Source: CAD feature listing. Evaluate the final solid. Frame: model axes, mm. A direction names the side the tool comes from. Coordinates: 2 decimals unless noted, no trailing zeros. Order: outer loops, then holes, each group sorted by start corner. A loop starts at its lowest first (then second) coordinate and runs counter-clockwise, first axis right, second up.
```python
from build123d import *

# Parameters (mm, degrees)
SKETCH2_W                      = 198.000030872
SKETCH2_H                      = 103.32125718
CUT_EXTRUDE1_DEPTH             = 3.6
FILLET1_R                      = 5
FILLET2_R                      = 3
F_4_CLEARANCE_HOLE1_AT_2_COUNT = 2
F_4_CLEARANCE_HOLE1_AT_2_PITCH = 13
CIRPATTERN1_COUNT              = 4
CIRPATTERN1_ANGLE              = 165
CUT_EXTRUDE2_DEPTH             = 3.6000001


with BuildPart() as part:
    # Sketch1 → Revolve1 (revolve)
    with BuildSketch(Plane(origin=(0, 0, 0), x_dir=(0, 0, -1), z_dir=(1, 0, 0)), mode=Mode.PRIVATE) as revolve1_sk:
        Polygon((0, 22), (0, 63), (1.5, 63), (1.5, 35), (2.6, 32.5), (2.6, 22), align=None)
    revolve(revolve1_sk.sketch.rotate(Axis((0, 0, 0), (0, 0, -1)), 90), axis=Axis((0, 0, 0), (0, 0, -1)))  # turned: the seam where the file's is

    # Sketch2 → Cut-Extrude1 (cut, through all)
    with BuildSketch(Plane.XY):
        with Locations((-0.69062002, -48.66062859)):
            Rectangle(SKETCH2_W, SKETCH2_H)
    extrude(amount=-CUT_EXTRUDE1_DEPTH, mode=Mode.SUBTRACT)

    # Fillet1
    fillet1_edges = [part.edges().sort_by_distance(p)[0] for p in [
        (0, 32.5, -2.6),
        (0, 35, -1.5),
    ]]
    fillet(fillet1_edges, radius=FILLET1_R)

    # Fillet2
    fillet2_edges = [part.edges().sort_by_distance(p)[0] for p in [
        (-21.794494718, 3, -1.3),
        (-62.92853089, 3, -0.75),
        (21.794494718, 3, -1.3),
        (62.92853089, 3, -0.75),
    ]]
    fillet(fillet2_edges, radius=FILLET2_R)

    # Sketch3 → #4 Clearance Hole1 (revolve, cut)
    with BuildSketch(Plane(origin=(-59.486691682, 7.831571533, 0), x_dir=(0, -1, 0), z_dir=(1, 0, 0))):
        Polygon((0, 0), (0, 136.775187864), (1.4732, 135.89), (1.4732, 0), align=None)
    f_4_clearance_hole1 = revolve(axis=Axis((-59.486691682, 7.831571533, 6.35), (0, 0, -1)), mode=Mode.SUBTRACT)

    # #4 Clearance Hole1 at 2: #4 Clearance Hole1 ×2
    with Locations(*[Vector(0.991444861, -0.130526192, 0) * (i * F_4_CLEARANCE_HOLE1_AT_2_PITCH) for i in range(1, F_4_CLEARANCE_HOLE1_AT_2_COUNT)]):
        add(f_4_clearance_hole1, mode=Mode.SUBTRACT)

    # CirPattern1: #4 Clearance Hole1 ×4 about axis
    cirpattern1_axis = Axis((0, 0, 0), (0, 0, -1))
    for i in range(1, CIRPATTERN1_COUNT):
        add(f_4_clearance_hole1.rotate(cirpattern1_axis, i * CIRPATTERN1_ANGLE / (CIRPATTERN1_COUNT - 1)), mode=Mode.SUBTRACT)

    # CirPattern1 copy 1 sketch → CirPattern1 copy 1 (revolve, cut)
    with BuildSketch(Plane(origin=(-21.702184822, 41.689509159, 0), x_dir=(-0.819152044, -0.573576436, 0), z_dir=(0.573576436, -0.819152044, 0))):
        Polygon((0, 0), (0, 136.775187864), (1.4732, 135.89), (1.4732, 0), align=None)
    revolve(axis=Axis((-21.702184822, 41.689509159, 6.35), (0, 0, -1)), mode=Mode.SUBTRACT)

    # CirPattern1 copy 2 sketch → CirPattern1 copy 2 (revolve, cut)
    with BuildSketch(Plane(origin=(21.702184822, 41.689509159, 0), x_dir=(-0.939692621, 0.342020143, 0), z_dir=(-0.342020143, -0.939692621, 0))):
        Polygon((0, 0), (0, 136.775187864), (1.4732, 135.89), (1.4732, 0), align=None)
    revolve(axis=Axis((21.702184822, 41.689509159, 6.35), (0, 0, -1)), mode=Mode.SUBTRACT)

    # CirPattern1 copy 3 sketch → CirPattern1 copy 3 (revolve, cut)
    with BuildSketch(Plane(origin=(46.597908485, 6.134731034, 0), x_dir=(-0.258819045, 0.965925826, 0), z_dir=(-0.965925826, -0.258819045, 0))):
        Polygon((0, 0), (0, 136.775187864), (1.4732, 135.89), (1.4732, 0), align=None)
    revolve(axis=Axis((46.597908485, 6.134731034, 6.35), (0, 0, -1)), mode=Mode.SUBTRACT)

    # Sketch5 → Cut-Extrude2 (cut, through all)
    with BuildSketch(Plane.XY):
        with BuildLine():
            Line((-4.5, 55), (4.5, 55))
            ThreePointArc((4.5, 55), (6.5, 53), (4.5, 51))
            Line((4.5, 51), (-4.5, 51))
            ThreePointArc((-4.5, 51), (-6.5, 53), (-4.5, 55))
        make_face()
    extrude(amount=-CUT_EXTRUDE2_DEPTH, mode=Mode.SUBTRACT)


solid = part.part
```
1. Material intervals for line 1 along Z through (x, y) = (-24.5, 33); line 2 along X through (y, z) = (12, -1.1); line 3 along Y through (x, z) = (-5.5, -0.5), sorted ascending.
2. Section query A-A, the plane y = 37.5. Output: boundary loops of the cut face in (x, z), plus the area to 3 significant figures.
3. Contact query for flat-ended pins moving along their axis: P1, Ø2.5, axis at x = -21.7, y = 41.69, coming from the +Z side; P2, Ø1.5, axis at x = 44, y = 20, coming from the -Z side; P3, Ø12, axis at x = -2.5, y = 41, coming from the -Z side. Output: stop coordinate, or through.
4. Draft query along X for faces 4 (the cylindrical face through (-1.297, 62.987, -0.76)), 5 (the flat face through (-38, 3, -1)), 6 (the cylindrical face through (58.05, 8.15, -0.74)). Return one class per face: +X half, -X half, draft (parallel to the pull), parting line (faces both ways), or undercut.
5. Access query for faces 1 (the flat face through (-1, 39, -1.5)), 2 (the cylindrical face through (-22.44, 3.62, -1.28)), 3 (the cylindrical face through (-45.16, 6.45, -0.74)). Directions: +Z, -Z, +X, -X, +Y, -Y. A direction counts if a zero-diameter tool reaches every point of the face in a straight line with its end or side. Return the directions, or none.
6. Section query B-B, the plane x = -49.5. Output: boundary loops of the cut face in (y, z), plus the area to 3 significant figures.
Answer key:
1. line 1: z = -1.5 to 0
1. line 2: x = -61.85 to -18.44, 18.44 to 61.85
1. line 3: y = 21.3 to 51.27, 54.73 to 62.76
2. outline: (-50.62, -1.5) - (50.62, -1.5) - (50.62, 0) - (-50.62, 0) - close
2. area: 152 mm2
3. P1: passes through
3. P2: stops at z = -1.5
3. P3: stops at z = -1.6
4. face 4: parting line
4. face 5: draft
4. face 6: undercut
5. face 1: -Z, +Y
5. face 2: +Z, -Z, -Y
5. face 3: +Z, -Z
6. outline: (3, -1.5) - (38.97, -1.5) - (38.97, 0) - (3, 0) - close
6. area: 54.0 mm2
